```python
from build123d import *

# Parameters (mm, degrees)
CROQUIS1_R              = 11
CROQUIS1_R_2            = 5.5
CROQUIS1_R_3            = 1.5
SALIENTE_EXTRUIR1_DEPTH = 4
SALIENTE_EXTRUIR2_DEPTH = 10
CORTAR_EXTRUIR1_REACH   = 44.247
CROQUIS3_R              = 1.75
REDONDEO1_R             = 5


with BuildPart() as part:
    # Croquis1 → Saliente-Extruir1 (new body)
    with BuildSketch(Plane(origin=(0, 0, 0), x_dir=(1, 0, 0), z_dir=(0, 1, 0))):
        with Locations(Location((0, 0, 0), (0, 0, 270))):
            Circle(CROQUIS1_R)
        with Locations(Location((0, 0, 0), (0, 0, 270))):
            Circle(CROQUIS1_R_2, mode=Mode.SUBTRACT)
        with Locations(Location((-8, 0, 0), (0, 0, 270))):
            Circle(CROQUIS1_R_3, mode=Mode.SUBTRACT)
        with Locations(Location((0, 8, 0), (0, 0, 270))):
            Circle(CROQUIS1_R_3, mode=Mode.SUBTRACT)
        with Locations(Location((8, 0, 0), (0, 0, 270))):
            Circle(CROQUIS1_R_3, mode=Mode.SUBTRACT)
        with Locations(Location((0, -8, 0), (0, 0, 270))):
            Circle(CROQUIS1_R_3, mode=Mode.SUBTRACT)
    extrude(amount=SALIENTE_EXTRUIR1_DEPTH)

    # Croquis2 → Saliente-Extruir2 (add)
    with BuildSketch(Plane(origin=(0, 4, 0), x_dir=(1, 0, 0), z_dir=(0, 1, 0))):
        with BuildLine():
            Line((2.680997215, 4.802317559), (27.429734557, 29.5510549))
            Line((27.429734557, 29.5510549), (29.5510549, 27.429734557))
            Line((29.5510549, 27.429734557), (4.802317559, 2.680997215))
            ThreePointArc((4.802317559, 2.680997215), (3.893730418, 3.893730418), (2.680997215, 4.802317559))
        make_face()
    extrude(amount=-SALIENTE_EXTRUIR2_DEPTH)

    # Croquis3 → Cortar-Extruir1 (cut, up to next)
    with BuildSketch(Plane(origin=(-1.060660172, 0, -1.060660172), x_dir=(-0.7071067811865465, 0, 0.7071067811865486), z_dir=(-0.7071067811865486, 0, -0.7071067811865465)), mode=Mode.PRIVATE) as cortar_extruir1_sk1:
        with Locations((-31.441502622, -1)):
            Circle(CROQUIS3_R)
    cortar_extruir1_tool1 = extrude(cortar_extruir1_sk1.sketch, amount=-CORTAR_EXTRUIR1_REACH, mode=Mode.PRIVATE) & part.part
    add(cortar_extruir1_tool1.solids().sort_by_distance((21.17184, -1, -23.29316))[0], mode=Mode.SUBTRACT)

    # Redondeo1
    redondeo1_edges = [part.edges().sort_by_distance(p)[0] for p in [
        (3.893730418, -6, -3.893730418),
        (28.490394728, -6, -28.490394728),
        (28.490394728, 4, -28.490394728),
    ]]
    fillet(redondeo1_edges, radius=REDONDEO1_R - 0.0001)  # a hair under: the kernel refuses the full size


solid = part.part
```
Input: part model. Units: mm. Frame: model coordinates. Round coordinates to 2 decimals unless told otherwise and drop trailing zeros. Loops run counter-clockwise (first coordinate to the right, second up) from the corner with the lowest first, then second, coordinate; pieces in that order, holes last.
1) Pin query (flat end, axial travel): pin 1 (4 mm diameter, centred on x = 8, z = 0, fed in from -Y); pin 2 (2 mm diameter, centred on y = 3, z = -9, fed in from -X); pin 3 (1.7 mm diameter, centred on x = 4, z = -3.5, fed in from -Y). Return the tip coordinate at first contact, or that it passes through.
Ans:
pin 1: stops at y = 0
pin 2: stops at x = -7.55
pin 3: stops at y = -3.48
2) Section query D-D on z = 7. Return the cut outline in (x, y).
Ans:
outline: (-8.49, 0) - (-1.12, 0) - (-1.12, 4) - (-8.49, 4) - close; (1.12, 0) - (8.49, 0) - (8.49, 4) - (1.12, 4) - close
3) Section query C-C on x = -8. Return the cut outline in (y, z).
Ans:
outline: (0, -7.55) - (4, -7.55) - (4, -1.5) - (0, -1.5) - close; (0, 1.5) - (4, 1.5) - (4, 7.55) - (0, 7.55) - close
4) Material intervals for line 1 (X direction, y = 1.8, z = 0); line 2 (X direction, y = 1.5, z = -9); line 3 (X direction, y = 0.5, z = -3.5), sorted ascending.
Ans:
line 1: x = -11 to -9.5, -6.5 to -5.5, 5.5 to 6.5, 9.5 to 11
line 2: x = -6.32 to -1.12, 1.12 to 6.32, 6.88 to 11.12
line 3: x = -10.43 to -4.24, 4.24 to 10.43
5) Pull-direction query (X, two-part tool) for faces 1 (the cylindrical face through (3.91, -0.49, -3.88)), 2 (the cylindrical face through (6.536, 1.972, -0.325)), 3 (the cylindrical face through (27.497, -4.496, -27.467)), 4 (the cylindrical face through (0.07, 1.97, -9.5)); classes: released by +X, released by -X, zero draft, split by the parting line, or undercut.
Ans:
face 1: released by -X
face 2: undercut
face 3: released by +X
face 4: undercut
6) Section query B-B on y = 1.5. Return the cut outline in (x, z).
Ans:
outline: (6.64, -8.77) - (26.96, -29.08) - (29.08, -26.96) - (8.77, -6.64) arc R11 ccw (long way) to start; hole circle Ø3 at (-8, 0); hole circle Ø11 at (0, 0); hole circle Ø3 at (0, -8); hole circle Ø3 at (0, 8); hole circle Ø3 at (8, 0)
7) Section query A-A on z = 0. Return the cut outline in (x, y).
Ans:
outline: (-11, 0) - (-9.5, 0) - (-9.5, 4) - (-11, 4) - close; (-6.5, 0) - (-5.5, 0) - (-5.5, 4) - (-6.5, 4) - close; (5.5, 0) - (6.5, 0) - (6.5, 4) - (5.5, 4) - close; (9.5, 0) - (11, 0) - (11, 4) - (9.5, 4) - close
